Autodesk Inventor part; units mm, degrees
ref_plane "YZ Plane" through (0, 0, 0) normal (1, 0, 0) x (0, 1, 0)
ref_plane "XZ Plane" through (0, 0, 0) normal (0, 1, 0) x (-1, 0, 0)
ref_plane "XY Plane" through (0, 0, 0) normal (0, 0, 1) x (1, 0, 0)
sketch "Esquisse1" plane through (0, 0, 0) normal (0, 1, 0) x (-1, 0, 0)
  line L0 (0, 0) -> (32, 0) construction
  line L1 (32, 0) -> (16, 27.7128) construction
  line L2 (16, 27.7128) -> (0, 0) construction
  line L3 (-17.9982, -10.3913) -> (15.6322, 9.0252) construction
  line L4 (11.2583, 6.5) -> (7.2583, 13.4282) construction
  line L5 (11.2583, 6.5) -> (-19.9186, -11.5) construction
  line L6 (-19.9186, -11.5) -> (-26.6686, 0.1913) construction
  line L7 (-26.6686, 0.1913) -> (-21.0394, 3.4413) construction
  line L8 (-21.0394, 3.4413) -> (-14.1112, 7.4413) construction
  line L9 (-14.1112, 7.4413) -> (-7.183, 11.4413) construction
  line L10 (-7.183, 11.4413) -> (-0.2548, 15.4413) construction
  circle A0 centre (-14.1112, 7.4413) radius 1 construction
  circle A1 centre (-7.183, 11.4413) radius 1
  circle A2 centre (-0.2548, 15.4413) radius 1
  circle A3 centre (7.2583, 13.4282) radius 1
  circle A4 centre (-21.0394, 3.4413) radius 1 construction
  circle A5 centre (-0.6112, -15.9413) radius 1 construction
  circle A6 centre (6.317, -11.9413) radius 1
  circle A7 centre (13.2452, -7.9413) radius 1
  circle A8 centre (15.2583, -0.4282) radius 1
  circle A9 centre (-7.5394, -19.9413) radius 1 construction
  circle A10 centre (-19.9186, -11.5) radius 11.6 construction
  line L11 (32, 0) -> (38.9282, 4) construction
  line L12 (36.0415, 0) -> (34.0207, -3.5) construction
  line L13 (34.0207, -3.5) -> (29.9793, -3.5) construction
  line L14 (29.9793, -3.5) -> (27.9585, 0) construction
  line L15 (27.9585, 0) -> (29.9793, 3.5) construction
  line L16 (29.9793, 3.5) -> (34.0207, 3.5) construction
  line L17 (34.0207, 3.5) -> (36.0415, 0) construction
  line L18 (34.0207, 3.5) -> (34.0207, -3.5) construction
  circle A11 centre (16, 27.7128) radius 2
  circle A12 centre (32, 0) radius 2
  line L19 (32, 0) -> (38.9282, 4) construction
  circle A13 centre (0, 0) radius 2
  line L20 (0, 0) -> (11.2583, 6.5) construction
  line L21 (-15.5131, 15.8695) -> (20.1782, 36.476)
  line L22 (20.1782, 36.476) -> (41.6782, -0.7631)
  line L23 (41.6782, -0.7631) -> (5.9869, -21.3695)
  line L24 (-7.183, 11.4413) -> (-11.183, 18.3695) construction
  line L25 (6.317, -11.9413) -> (10.317, -18.8695) construction
  line L26 (6.317, -11.9413) -> (1.9869, -14.4413) construction
  line L27 (-15.5131, 15.8695) -> (5.9869, -21.3695)
  dimension "d0" = 32
  dimension "d1" = 32
  dimension "d2" = 60
  dimension "d4" = 8
  dimension "d6" = 36
  dimension "d7" = 13.5
  dimension "d8" = 6.5
  dimension "d9" = 8
  dimension "d10" = 8
  dimension "d11" = 8
  dimension "d13" = 2
  dimension "d14" = 11.6
  dimension "d15" = 8
  dimension "d16" = 7
  dimension "d17" = 4
  dimension "d19" = 8
  dimension "d69" = 210
  dimension "d70" = 13
  dimension "d83" = 8
  dimension "d84" = 8
  dimension "d85" = 5
extrude "Extrusion7" add sketch "Esquisse1" along normal blind 12
sketch "Esquisse9" plane through (0, 0, 0) normal (0, -1, 0) x (1, 0, 0)
  circle A0 centre (0, 0) radius 2
  circle A1 centre (-32, 0) radius 2
  circle A2 centre (-16, 27.7128) radius 2
  line L0 (-41.6782, -0.7631) -> (-5.9869, -21.3695)
  line L1 (18.1112, 14.3695) -> (-3.3888, -22.8695)
  line L2 (15.5131, 15.8695) -> (-20.1782, 36.476)
  line L3 (-19.5, 25.6921) -> (-19.5, 29.7335)
  line L4 (-19.5, 29.7335) -> (-16, 31.7543)
  line L5 (-16, 31.7543) -> (-12.5, 29.7335)
  line L6 (-12.5, 29.7335) -> (-12.5, 25.6921)
  line L7 (-12.5, 25.6921) -> (-16, 23.6714)
  line L8 (-16, 23.6714) -> (-19.5, 25.6921)
  line L9 (-28.5, 2.0207) -> (-28.5, -2.0207)
  line L10 (-28.5, -2.0207) -> (-32, -4.0415)
  line L11 (-32, -4.0415) -> (-35.5, -2.0207)
  line L12 (-35.5, -2.0207) -> (-35.5, 2.0207)
  line L13 (-35.5, 2.0207) -> (-32, 4.0415)
  line L14 (-32, 4.0415) -> (-28.5, 2.0207)
  line L15 (-19.5, 25.6921) -> (-12.5, 25.6921) construction
  line L16 (4.0415, 0) -> (2.0207, -3.5)
  line L17 (2.0207, -3.5) -> (-2.0207, -3.5)
  line L18 (-2.0207, -3.5) -> (-4.0415, 0)
  line L19 (-4.0415, 0) -> (-2.0207, 3.5)
  line L20 (-2.0207, 3.5) -> (2.0207, 3.5)
  line L21 (2.0207, 3.5) -> (4.0415, 0)
  point P0 (-3.3888, -22.8695)
  dimension "d75" = 7
fillet "Congé15" radius 8 1 edges at (-41.6782, 6, -0.7631)
fillet "Congé16" radius 8 1 edges at (-20.1782, 6, 36.476)
extrude "Extrusion8" cut sketch "Esquisse9" against normal blind 3
fillet "Congé17" radius 10 1 edges at (15.5131, 6, 15.8695)
fillet "Congé18" radius 10 1 edges at (-5.9869, 6, -21.3695)
properties part number "joint3+ax12imprint_v3"
Design review of the part built by this model. Coordinates are the model's own, in mm. A direction names the side the tool comes from. Give positions to 0.01 mm unless a question says otherwise; leave off trailing zeros. Write each loop counter-clockwise with the first axis right and the second up, starting at its lowest first coordinate (ties: lowest second). Pieces come first, ordered by that corner, then holes. Notation, with made-up numbers: (81.5, 25.25) -> (95.5, 25.25) arc R31 ccw to (95.5, 54.25) -> close; hole circle Ø6 at (12.5, 58.5). An arc over 180 degrees is marked (long way). Answer in a Markdown table with one row per item.
(1) Consider section B-B (y = 5). Count the separate pieces of the cut face and the enclosed holes in it, then the cut area to 3 significant figures.
Results:
| item | result |
|---|---|
| separate pieces | 1 |
| enclosed holes | 9 |
| area | 1,650 mm2 |
(2) Clearance check with flat-ended pins moving along their axes: pin 1 (1.5 mm diameter, centred on x = -14.5, y = 6, fed in from -Z); pin 2 (3.5 mm diameter, centred on y = 1, z = -0.5, fed in from +X); pin 3 (1.5 mm diameter, centred on x = -21.5, y = 1.5, fed in from +Z). State where each tip first meets the part, or that it passes through.
Results:
| item | result |
|---|---|
| pin 1 | z = -16.83 |
| pin 2 | x = 7.07 |
| pin 3 | z = 32.74 |
(3) Consider section C-C (z = 9). State the section outline as (x, y) points.
Results:
| item | result |
|---|---|
| outline | (-36.04, 0) -> (11.32, 0) -> (11.32, 12) -> (-36.04, 12) -> close |
(4) Mouldability with a two-part tool opening along X and no side actions: class faces 3 (the flat face through (-13, 0, 8)), 4 (the flat face through (-3.058, 5.916, 26.591)), 5 (the flat face through (-30.834, 5.916, 18.02)), 6 (the flat face through (-30.274, 1.479, 3.045)) as +X half, -X half, draft (parallel to the pull), parting line (faces both ways), or undercut.
Results:
| item | result |
|---|---|
| face 3 | draft |
| face 4 | +X half |
| face 5 | -X half |
| face 6 | undercut |
(5) Consider section D-D (z = 22.5). State the section outline as (x, y) points, then the cut area to 3 significant figures.
Results:
| item | result |
|---|---|
| outline | (-28.25, 0) -> (4.03, 0) -> (4.03, 12) -> (-28.25, 12) -> close |
| area | 387 mm2 |
(6) Consider section A-A (x = 0). State the section outline as (y, z) points, then the cut area to 3 significant figures.
Results:
| item | result |
|---|---|
| outline | (0, -11) -> (12, -11) -> (12, -2) -> (3, -2) -> (3, -3.5) -> (0, -3.5) -> close; (0, 3.5) -> (3, 3.5) -> (3, 2) -> (12, 2) -> (12, 14.47) -> (0, 14.47) -> close; (0, 16.41) -> (12, 16.41) -> (12, 24.83) -> (0, 24.83) -> close |
| area | 350 mm2 |
(7) For faces 1 (the flat face through (-3.045, 1.479, 1.726)), 2 (the cylindrical face through (0, 7, 2)), list the 3-axis set-ups (+Z, -Z, +X, -X, +Y, -Y) from which the entire face can be reached by the end or side of a thin tool; tool diameter is ignored.
Results:
| item | result |
|---|---|
| face 1 | -Y |
| face 2 | +Y, -Y |
(8) To check wall thickness, follow probe 1 along X at (y, z) = (7.75, 0); probe 2 along X at (y, z) = (1.5, 3); probe 3 along Z at (x, y) = (0, 6.5). State the ranges of each line that lie inside material, in increasing order.
Results:
| item | result |
|---|---|
| probe 1 | -38.45 to -34, -30 to -16.16, -14.35 to -2, 2 to 6.35 |
| probe 2 | -38.71 to -33.8, -30.2 to -2.31, 2.31 to 8.08 |
| probe 3 | -11 to -2, 2 to 14.47, 16.41 to 24.83 |
